Geometry check sheet. Reference: the model listing, model coordinates, mm. Face numbers are marked on the shaded views. Round coordinates to 2 decimals unless told otherwise and drop trailing zeros. Loops run counter-clockwise (first coordinate to the right, second up) from the corner with the lowest first, then second, coordinate; pieces in that order, holes last.
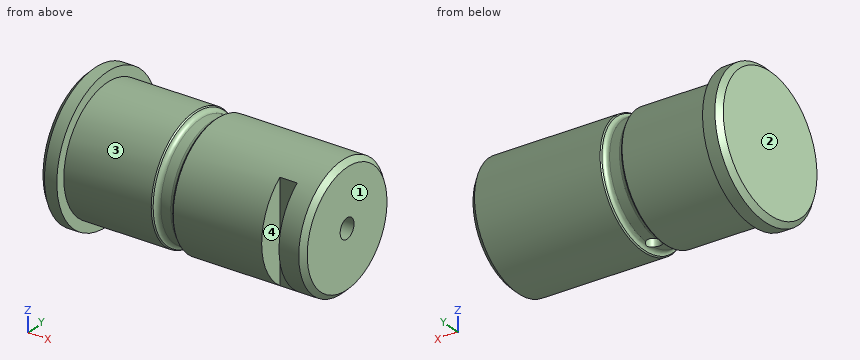
```python
from build123d import *

# Parameters (mm, degrees)
F0_R      = 25
F1_DEPTH  = 97
F2_SIZE   = 2
F3_R      = 29
F4_DEPTH  = 7
F5_SIZE   = 2
F8_W      = 7
F8_H      = 14.5
F9_DEPTH  = 50
F11_D     = 8
F11_DEPTH = 65
F11_TIP   = 2.4034424761
F13_D     = 6
F13_DEPTH = 29.001


# Not quite as in the source:
# - a fillet or chamfer that OpenCascade refuses, or shapes differently, is made with other operations: its cross-section is extruded or revolved along the edge and cut away or added


with BuildPart() as f1:
    # F0 (on Right) → F1 (new body)
    with BuildSketch(Plane.YZ):
        Circle(F0_R)
    extrude(amount=F1_DEPTH)

    # F2
    f2_edges = [f1.edges().sort_by_distance(p)[0] for p in [
        (97, -25, 0),
    ]]
    chamfer(f2_edges, length=F2_SIZE)

    # F3 (on Right) → F4 (join)
    with BuildSketch(Plane.YZ):
        Circle(F3_R)
    extrude(amount=-F4_DEPTH)

    # F5
    f5_edges = [f1.edges().sort_by_distance(p)[0] for p in [
        (-7, -29, 0),
    ]]
    chamfer(f5_edges, length=F5_SIZE)

    # F6 (on Top) → F7 (revolve, cut)
    with BuildSketch(Plane.XY):
        with BuildLine():
            Line((43.7990407646, 27), (35.7990407646, 27))
            Line((35.7990407646, 27), (35.7990407646, 25))
            ThreePointArc((35.7990407646, 25), (36.3848272022, 23.5857864376), (37.7990407646, 23))
            Line((37.7990407646, 23), (41.7990407646, 23))
            ThreePointArc((41.7990407646, 23), (43.2132543269, 23.5857864376), (43.7990407646, 25))
            Line((43.7990407646, 25), (43.7990407646, 27))
        make_face()
    revolve(axis=Axis((58.3793800324, 0, 0), (1, 0, 0)), mode=Mode.SUBTRACT)

    # F8 (on Top) → F9 (cut, symmetric)
    with BuildSketch(Plane.XY):
        with Locations((83.5, -21.75)):
            Rectangle(F8_W, F8_H)
    extrude(amount=F9_DEPTH, both=True, mode=Mode.SUBTRACT)

    # F11
    with Locations(Plane.YZ.offset(97)):
        with Locations((0, 0)):
            Hole(F11_D / 2, depth=F11_DEPTH)
            with Locations((0, 0, -(F11_DEPTH + F11_TIP / 2))):  # 118° drill point
                Cone(0, F11_D / 2, F11_TIP, mode=Mode.SUBTRACT)

    # F13 (through all, one way)
    with BuildSketch(Plane.XY):
        with Locations((39.7990407646, 0)):
            Circle(F13_D / 2)
    extrude(amount=-F13_DEPTH, mode=Mode.SUBTRACT)

    # F14: chamfer of 0.5 on 2 edges, made by hand

    # F14_s1 → F14_t2 (revolve, cut)
    with BuildSketch(Plane.XY):
        with BuildLine():
            Line((35.3495510218, 25), (35.8394489703, 24.6))
            ThreePointArc((35.8394489703, 24.6), (35.8098979776, 24.7918871147), (35.7990407646, 25))
            Line((35.7990407646, 25), (35.3495510218, 25))
        make_face()
    revolve(axis=Axis((35.7990407646, 0, 0), (1, 0, 0)), mode=Mode.SUBTRACT)

    # F14_s3 → F14_t4 (revolve, cut)
    with BuildSketch(Plane.XY):
        with BuildLine():
            Line((43.7586325588, 24.6), (44.2485305074, 25))
            Line((44.2485305074, 25), (43.7990407646, 25))
            ThreePointArc((43.7990407646, 25), (43.7881835515, 24.7918871147), (43.7586325588, 24.6))
        make_face()
    revolve(axis=Axis((43.7990407646, 0, 0), (1, 0, 0)), mode=Mode.SUBTRACT)


solid = f1.part
```
1) Sectioned sample at A-A, the plane x = 90.5. Record the cut outline in (y, z), then the cut area to 3 significant figures.
Report:
outline: circle Ø50 at (0, 0); hole circle Ø8 at (0, 0)
area: 1,910 mm2
2) Mould release check, pull along X, two halves, no side actions. Record for the marked faces 1, 2, 3 and 4: +X half, -X half, draft (parallel to the pull), parting line (faces both ways), or undercut.
Report:
face 1: +X half
face 2: -X half
face 3: draft
face 4: undercut
3) Gauge pin test, flat ends, axial feed: pin 1 (12 mm diameter, centred on x = 70.5, z = -6, fed in from +Y); pin 2 (3 mm diameter, centred on x = 46.5, z = 23, fed in from +Y); pin 3 (2 mm diameter, centred on x = 48, z = -10.5, fed in from -Y); pin 4 (13 mm diameter, centred on y = 0, z = 0, fed in from +X). Record the tip position at first contact, or that the pin passes through.
Report:
pin 1: stops at y = 25
pin 2: stops at y = 12.76
pin 3: stops at y = -23.12
pin 4: stops at x = 97
4) Scan lines: line 1 along Z through (x, y) = (70, 0); line 2 along Y through (x, z) = (82, 0); line 3 along X through (y, z) = (-18.5, -10.5). Record each from-to range of solid material in increasing order.
Report:
line 1: z = -25 to -4, 4 to 25
line 2: y = -14.5 to -4, 4 to 25
line 3: x = -7 to 80, 87 to 97
